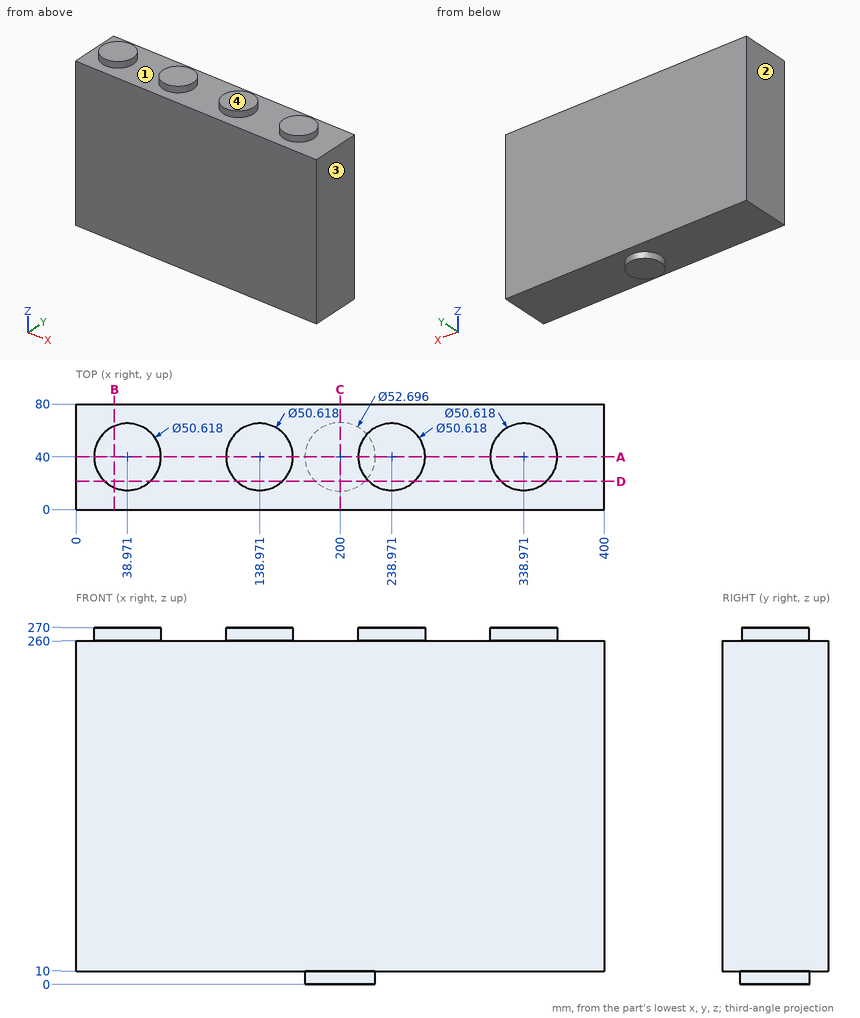
Input: dimensioned drawing with shaded views. Units: mm. Origin: part minimum x, y, z. Round coordinates to 2 decimals unless told otherwise and drop trailing zeros. Loops run counter-clockwise (first coordinate to the right, second up) from the corner with the lowest first, then second, coordinate; pieces in that order, holes last. Notation, with made-up numbers: (36, 41.25) -> (69, 41.25) arc R37 ccw to (69, 80.25) -> close; hole circle Ø3 at (76.25, -12). An arc over 180 degrees is marked (long way). Answer as a JSON object with one key per item and string values. Group by question number.
Q1. Section query C-C (x = 200). Output: boundary loops of the cut face in (y, z), plus the area to 3 significant figures.
Q2. Mould query, pull axis X, two halves, no side actions, for the marked faces 1, 2, 3 and 4. Classes: pulls with the +X half, pulls with the -X half, needs draft (parallel to the pull), parting line crosses it, or undercut.
Q3. Section query D-D (y = 21.5). Output: boundary loops of the cut face in (x, z).
Q4. Section query B-B (x = 29). Output: boundary loops of the cut face in (y, z).
Q5. Section query A-A (y = 40). Output: boundary loops of the cut face in (x, z), plus the area to 3 significant figures.
Q6. Ray query, line 1 (Z direction, x = 319, y = 63.5); line 2 (Z direction, x = 213, y = 55.5). Return the intervals inside material, ascending. Write a range as from..to.
Completed:
{
 "1": {"outline": "(0, 10) -> (13.65, 10) -> (13.65, 0) -> (66.35, 0) -> (66.35, 10) -> (80, 10) -> (80, 260) -> (0, 260) -> close", "area": "20,500 mm²"},
 "2": {"face 1": "undercut", "face 2": "pulls with the -X half", "face 3": "pulls with the +X half", "face 4": "needs draft"},
 "3": {"outline": "(0, 10) -> (181.24, 10) -> (181.24, 0) -> (218.76, 0) -> (218.76, 10) -> (400, 10) -> (400, 260) -> (356.24, 260) -> (356.24, 270) -> (321.7, 270) -> (321.7, 260) -> (256.24, 260) -> (256.24, 270) -> (221.7, 270) -> (221.7, 260) -> (156.24, 260) -> (156.24, 270) -> (121.7, 270) -> (121.7, 260) -> (56.24, 260) -> (56.24, 270) -> (21.7, 270) -> (21.7, 260) -> (0, 260) -> close"},
 "4": {"outline": "(0, 10) -> (80, 10) -> (80, 260) -> (63.26, 260) -> (63.26, 270) -> (16.74, 270) -> (16.74, 260) -> (0, 260) -> close"},
 "5": {"outline": "(0, 10) -> (173.65, 10) -> (173.65, 0) -> (226.35, 0) -> (226.35, 10) -> (400, 10) -> (400, 260) -> (364.28, 260) -> (364.28, 270) -> (313.66, 270) -> (313.66, 260) -> (264.28, 260) -> (264.28, 270) -> (213.66, 270) -> (213.66, 260) -> (164.28, 260) -> (164.28, 270) -> (113.66, 270) -> (113.66, 260) -> (64.28, 260) -> (64.28, 270) -> (13.66, 270) -> (13.66, 260) -> (0, 260) -> close", "area": "103,000 mm²"},
 "6": {"line 1": "10..260", "line 2": "0..260"}
}
